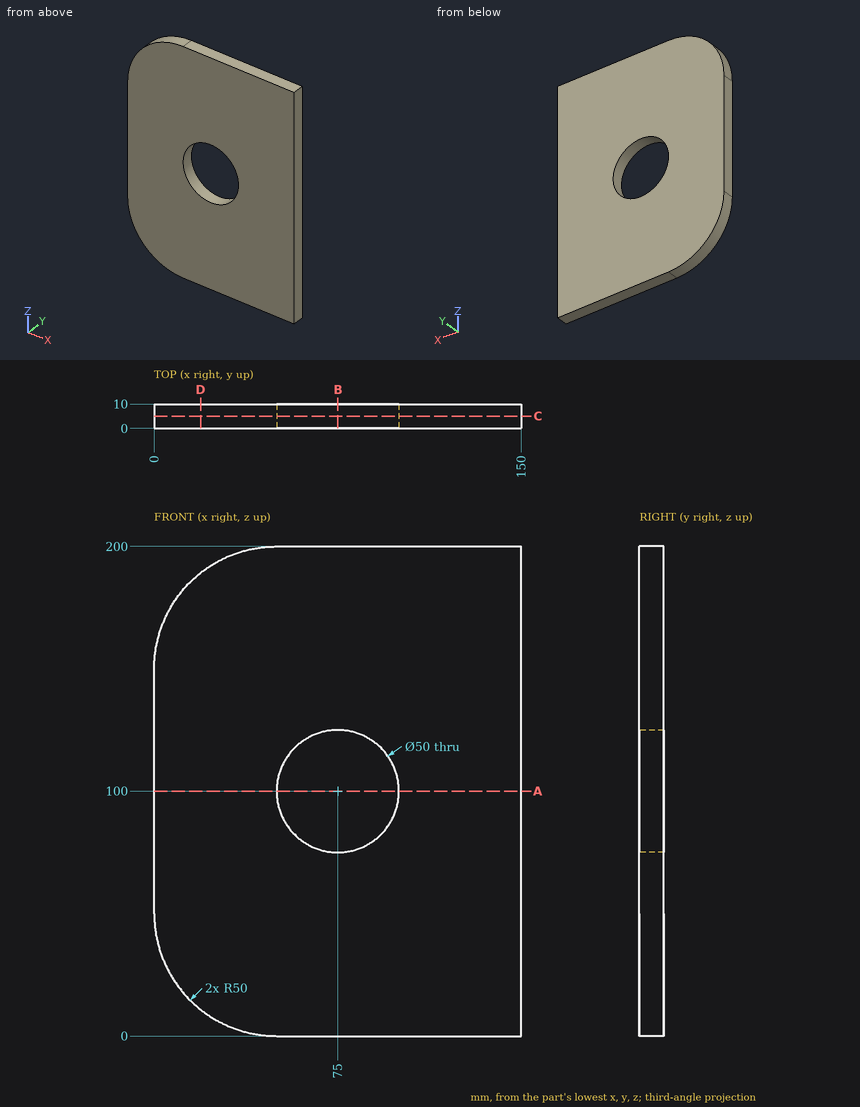
Input: dimensioned drawing with shaded views. Units: mm. Origin: part minimum x, y, z. Coordinates: 2 decimals unless noted, no trailing zeros. Order: outer loops, then holes, each group sorted by start corner. A loop starts at its lowest first (then second) coordinate and runs counter-clockwise, first axis right, second up. Notation, with made-up numbers: M 26,32.25 L 55,32.25 A13 ccw 55,45.25 Z; hole C 58,68 d8. An arc over 180 degrees is marked long. Write each question's results on one line, items separated by ' | '. Start each with the question number.
Item 1: Cut plane C-C (y = 5). Return loops of the section in (x, z), and give its area (3 significant figures).
Item 2: First-contact query: pin 1 Ø10 at (x, z) = (92, 84) entering from -Y. Flat tip, straight axial feed; report the tip coordinate or a pass-through.
Item 3: Cut plane A-A (z = 100). Return loops of the section in (x, y), and give its area (3 significant figures).
Item 4: Line query: probe 1 along Z at (x, y) = (75, 5.25); probe 2 along X at (y, z) = (3, 121); probe 3 along X at (y, z) = (9.75, 89). Output: solid intervals per line, ascending.
Item 5: Cut plane B-B (x = 75). Return loops of the section in (y, z).
Item 6: Cut plane D-D (x = 19). Return loops of the section in (y, z).
Checked values:
1) outline: M 0,50 A50 ccw 50,0 L 150,0 L 150,200 L 50,200 A50 ccw 0,150 Z; hole C 75,100 d50 | area: 27,000 mm2
2) pin 1: stops at y = 0
3) outline: M 0,0 L 50,0 L 50,10 L 0,10 Z; M 100,0 L 150,0 L 150,10 L 100,10 Z | area: 1,000 mm2
4) probe 1: z = 0 to 75, 125 to 200 | probe 2: x = 0 to 61.44, 88.56 to 150 | probe 3: x = 0 to 52.55, 97.45 to 150
5) outline: M 0,0 L 10,0 L 10,75 L 0,75 Z; M 0,125 L 10,125 L 10,200 L 0,200 Z
6) outline: M 0,10.77 L 10,10.77 L 10,189.23 L 0,189.23 Z
